Read the model definition and answer for the solid it produces. Units are mm, in the model's axes. A direction names the side the tool comes from. Give positions to 0.01 mm unless a question says otherwise; leave off trailing zeros. Loops run counter-clockwise (first coordinate to the right, second up) from the corner with the lowest first, then second, coordinate; pieces in that order, holes last. Notation, with made-up numbers: (-19, 74) - (-6, 74) arc R13 cw to (-6, 97) - close; hole circle Ø9 at (-31, -20). An arc over 180 degrees is marked (long way). Write each question's results on one line, items separated by ' | '. Start each with the question number.
Q1. Given pin 1 (3 mm diameter, centred on x = 21.5, z = 7, fed in from +Y); pin 2 (7 mm diameter, centred on x = -21.48, z = 10, fed in from +Y); pin 3 (1.5 mm diameter, centred on x = -20, z = 6, fed in from -Y), each flat-ended and moving along its own axis, determine where each tip first touches the part or whether it passes through.
Q2. The part is cut by section B-B, the plane z = 5. Write down the section's boundary in (x, y).
Q3. For faces 1 (the flat face through (-20.738, 1.386, 7.638)), 2 (the flat face through (25, 0, 6.25)), 3 (the flat face through (-21.555, 4.447, 7.638)), 4 (the flat face through (-21.555, -4.447, 7.638)), determine the directions among +Z, -Z, +X, -X, +Y, -Y from which every point of the face is accessible in a straight line to the end or side of a thin tool.
Q4. The part is cut by section D-D, the plane x = -22. Write down the section's boundary in (y, z), plus the area to 3 significant figures.
Q5. The part is cut by section C-C, the plane y = 14. Write down the section's boundary in (x, z), plus the area to 3 significant figures.
Q6. The part is cut by section A-A, the plane x = 0. Write down the section's boundary in (y, z), plus the area to 3 significant figures.
Q7. Determine the mould class of faces 5 (the flat face through (22, -2.5, 10)), 6 (the cylindrical face through (-19.434, -2.922, 10.646)), 7 (the flat face through (-14, 6, 20)) for opening direction Z: +Z half, -Z half, draft (parallel to the pull), parting line (faces both ways), or undercut.
Q8. Find the intervals of material crossed by line 1 (X direction, y = 0, z = 5); line 2 (Y direction, x = 0, z = 14.25); line 3 (X direction, y = -2.8, z = 10), in increasing order. Write a range as from..to.
```python
from build123d import *

# Parameters (mm, degrees)
PAD_DEPTH         = 20
SKETCH001_R       = 2.15
POCKET_DEPTH      = 17.001
POCKET_DEPTH_BACK = -17.001
PAD001_DEPTH      = 2.5


with BuildPart() as part:
    # Sketch → Pad (new body)
    with BuildSketch(Plane.XY):
        with BuildLine():
            ThreePointArc((-14.96663, -1), (15, 0), (-14.96663, 1))
            Line((-14.96663, 1), (-26.673727, 1.782213))
            Line((-26.673727, 1.782213), (-26.473727, 4.775539))
            Line((-26.473727, 4.775539), (-16.495974, 4.108873))
            ThreePointArc((-16.495974, -4.108873), (17, 0), (-16.495974, 4.108873))
            Line((-26.473727, -4.775539), (-16.495974, -4.108873))
            Line((-26.673727, -1.782213), (-26.473727, -4.775539))
            Line((-14.96663, -1), (-26.673727, -1.782213))
        make_face()
    extrude(amount=PAD_DEPTH)

    # Sketch001 → Pocket (cut, two sides)
    with BuildSketch(Plane.XZ) as pocket_sk:
        with Locations((-21.484851, 10)):
            Circle(SKETCH001_R)
    extrude(amount=-POCKET_DEPTH, mode=Mode.SUBTRACT)
    extrude(pocket_sk.sketch, amount=-POCKET_DEPTH_BACK, mode=Mode.SUBTRACT)

    # Sketch002 → Pad001 (join, symmetric)
    with BuildSketch(Plane.XZ):
        with BuildLine():
            Line((16.7, 20), (16.7, 0))
            Line((16.7, 0), (26.7, 0))
            Line((26.7, 0), (26.7, 3.75))
            Line((26.7, 3.75), (23.865064, 3.75))
            ThreePointArc((23.865064, 6.25), (19.2, 5), (23.865064, 3.75))
            Line((23.865064, 6.25), (26.7, 6.25))
            Line((26.7, 6.25), (26.7, 20))
            Line((26.7, 20), (16.7, 20))
        make_face()
    extrude(amount=PAD001_DEPTH, both=True)


solid = part.part
```
Check sheet entries:
1) pin 1: stops at y = 2.5 | pin 2: stops at y = 4.68 | pin 3: stops at y = -4.39
2) outline: (-26.67, -1.78) - (-26.47, -4.78) - (-16.5, -4.11) arc R17 ccw to (16.82, -2.5) - (19.2, -2.5) - (19.2, 2.5) - (16.82, 2.5) arc R17 ccw to (-16.5, 4.11) - (-26.47, 4.78) - (-26.67, 1.78) - (-14.97, 1) arc R15 cw (long way) to (-14.97, -1) - close
3) face 1: +Z, -Z, -X | face 2: +X, +Y, -Y | face 3: +Z, -Z, +Y | face 4: +Z, -Z, -Y
4) outline: (-4.48, 0) - (-1.47, 0) - (-1.47, 7.91) - (-4.48, 7.91) - close; (-4.48, 12.09) - (-1.47, 12.09) - (-1.47, 20) - (-4.48, 20) - close; (1.47, 0) - (4.48, 0) - (4.48, 7.91) - (1.47, 7.91) - close; (1.47, 12.09) - (4.48, 12.09) - (4.48, 20) - (1.47, 20) - close | area: 95.2 mm^2
5) outline: (-9.64, 0) - (-5.39, 0) - (-5.39, 20) - (-9.64, 20) - close; (5.39, 0) - (9.64, 0) - (9.64, 20) - (5.39, 20) - close | area: 170 mm^2
6) outline: (-17, 0) - (-15, 0) - (-15, 20) - (-17, 20) - close; (15, 0) - (17, 0) - (17, 20) - (15, 20) - close | area: 80.0 mm^2
7) face 5: draft | face 6: undercut | face 7: +Z half
8) line 1: x = 15..19.2 | line 2: y = -17..-15, 15..17 | line 3: x = -26.61..-23.63, -19.33..-14.74, 14.74..16.77
